The model under review builds one solid part; all positions refer to its coordinate system, in mm. A direction names the side the tool comes from. Round coordinates to 2 decimals unless told otherwise and drop trailing zeros. Order: outer loops, then holes, each group sorted by start corner. A loop starts at its lowest first (then second) coordinate and runs counter-clockwise, first axis right, second up. Notation, with made-up numbers: (85.25, 39.25) -> (106.25, 39.25) arc R12 cw to (106.25, 54.25) -> close; hole circle Ø6 at (10.5, 52). An arc over 180 degrees is marked (long way). Use a Markdown table: item, result. Add a question column.
Autodesk Inventor part; units mm, degrees
ref_plane "YZ Plane" through (0, 0, 0) normal (1, 0, 0) x (0, 1, 0)
ref_plane "XZ Plane" through (0, 0, 0) normal (0, 1, 0) x (-1, 0, 0)
ref_plane "XY Plane" through (0, 0, 0) normal (0, 0, 1) x (1, 0, 0)
sketch "Sketch1" plane through (0, 0, 0) normal (1, 0, 0) x (0, 1, 0)
  line L0 (0, 0) -> (100, 0)
  line L1 (100, 0) -> (100, -11)
  line L2 (100, -11) -> (0, -11)
  line L3 (0, -11) -> (0, 0)
  line L4 (60, -11) -> (40, -11)
  line L5 (40, -11) -> (40, -21)
  line L6 (40, -21) -> (60, -21)
  line L7 (60, -21) -> (60, -11)
  line L8 (0, -11) -> (100, -11)
  line L9 (100, -11) -> (100, -5)
  line L10 (100, -5) -> (0, -5)
  line L11 (0, -5) -> (0, -11)
  circle A0 centre (39, -12) radius 2.5
  line L12 (37.2322, -10.2322) -> (40.7678, -13.7678) construction
  circle A1 centre (61, -12) radius 2.5
  line L13 (62.7678, -10.2322) -> (59.2322, -13.7678) construction
  point P0 (0, -5)
  point P1 (60, -14.2913)
  point P2 (63.2913, -11)
  point P3 (36.7087, -11)
  point P4 (40, -14.2913)
  dimension "d1" = 11
  dimension "d2" = 100
  dimension "d3" = 10
  dimension "d4" = 20
  dimension "d5" = 40
  dimension "d7" = 6
  dimension "d31" = 5
  dimension "d32" = 45
  dimension "d33" = 1
  dimension "d34" = 1
  dimension "d35" = 5
  dimension "d36" = 45
  dimension "d37" = 1
  dimension "d38" = 1
revolve "Revolution1" add sketch "Sketch1" angle 360 about axis through (0, 0, 0) along (0, 1, 0) contours L10 L1 L2 A1 A0 L3 | L2 A1 L7 L6 L5 A0
sketch "Sketch2" plane through (0, 0, 0) normal (1, 0, 0) x (0, 1, 0)
  circle A0 centre (87, 0) radius 2
  line L0 (100, 11) -> (100, -11)
  point P0 (0, 0)
  dimension "d8" = 4
  dimension "d9" = 13
extrude "Extrusion1" cut sketch "Sketch2" along normal through all both and the other way through all
sketch "Sketch3" plane through (0, 0, 0) normal (0, 0, 1) x (1, 0, 0)
  circle A0 centre (0, 87) radius 2
  line L0 (-11, 100) -> (11, 100)
  point P0 (0, 0)
  dimension "d12" = 13
  dimension "d13" = 4
extrude "Extrusion2" cut sketch "Sketch3" against normal through all both and the other way through all
sketch "Sketch4" plane through (0, 0, 0) normal (0, -1, 0) x (1, 0, 0)
  circle A0 centre (0, 0) radius 9
  line L0 (-9, 0) -> (-11, 0)
  circle A1 centre (0, 0) radius 11
  line L1 (0, 9) -> (0, 11)
  line L2 (9, 0) -> (11, 0)
  line L3 (0, -9) -> (0, -11)
  line L4 (-4.5, -7.7942) -> (-5.5, -9.5263)
  line L5 (-7.7942, -4.5) -> (-9.5263, -5.5)
  line L6 (-7.7942, 4.5) -> (-9.5263, 5.5)
  line L7 (-4.5, 7.7942) -> (-5.5, 9.5263)
  line L8 (4.5, 7.7942) -> (5.5, 9.5263)
  line L9 (7.7942, 4.5) -> (9.5263, 5.5)
  line L10 (7.7942, -4.5) -> (9.5263, -5.5)
  line L11 (4.5, -7.7942) -> (5.5, -9.5263)
  dimension "d21" = 18
  dimension "d22" = 30
  dimension "d23" = 30
  dimension "d24" = 30
  dimension "d25" = 30
extrude "Extrusion3" cut sketch "Sketch4" against normal blind 30 contours A0 L9 A1 L2 | L10 A1 L11 A0 | A0 L1 A1 L8 | L3 A1 L4 A0 | A0 L6 A1 L7 | L5 A1 L0 A0
equation "\"d34\" = d33"
equation "\"d38\" = d37"
equation "\"d23\" = d22"
equation "\"d24\" = d22"
equation "\"d25\" = d22"
properties part number "shaft"
Q1. Mouldability with a two-part tool opening along X and no side actions: class faces 1 (the flat face through (14, 60, -4)), 2 (the cylindrical face through (0.923, 85.226, 7.836)), 3 (the cylindrical face through (-4.213, 81.389, -10.161)), 4 (the cylindrical face through (-6.34, 14.79, 6.39)) as pulls with the +X half, pulls with the -X half, needs draft (parallel to the pull), parting line crosses it, or undercut.
Q2. Add section C-C (y = 53). Write out the cut boundary in (x, z).
Q3. Add section B-B (y = 87). Write out the cut boundary in (x, z).
Q4. Add section A-A (y = 11.5). Write out the cut boundary in (x, z).
Q5. Wall thickness on line 1 (X direction, y = 36, z = 0); line 2 (Y direction, x = 6.75, z = 0); line 3 (Z direction, x = 19.5, y = 59): over which ranges is each line inside the solid? List them lowest first. Write a range as [from, to].
Q6. Machinability: for faces 5 (the cylindrical face through (-8.7, 14.8, -2.3)), 6 (the flat face through (0, 15, 10)), 7 (the flat face through (14, 40, -4)), 8 (the cylindrical face through (8.7, 14.8, 2.3)), which of the approach directions +Z, -Z, +X, -X, +Y, -Y give a long, thin tool a straight path to every point of the face, cutting with its end or side? Answer none if there is none.
Q7. Insertion check: pin 1 (3 mm diameter, centred on y = 87, z = 0, fed in from -X); pin 2 (1.6 mm diameter, centred on x = 9.5, y = 20.5, fed in from +Z); pin 3 (6 mm diameter, centred on x = -16, y = 43.5, fed in from +Z); pin 4 (0.6 mm diameter, centred on y = 12.5, z = -10, fed in from -X). Each pin has a flat end and moves straight along its axis. Give the tip position at first contact, or say it passes through.
Report:
| question | item | result |
|---|---|---|
| 1 | face 1 | needs draft |
| 1 | face 2 | undercut |
| 1 | face 3 | parting line crosses it |
| 1 | face 4 | undercut |
| 2 | outline | circle Ø42 at (0, 0); hole circle Ø10 at (0, 0) |
| 3 | outline | (-10.82, -2) arc R11 ccw to (-2, -10.82) -> (-2, -4.58) arc R5 cw to (-4.58, -2) -> close; (-10.82, 2) -> (-4.58, 2) arc R5 cw to (-2, 4.58) -> (-2, 10.82) arc R11 ccw to start; (2, -10.82) arc R11 ccw to (10.82, -2) -> (4.58, -2) arc R5 cw to (2, -4.58) -> close; (2, 4.58) arc R5 cw to (4.58, 2) -> (10.82, 2) arc R11 ccw to (2, 10.82) -> close |
| 4 | outline | (-11, 0) -> (-9, 0) arc R9 ccw to (-7.79, -4.5) -> (-9.53, -5.5) arc R11 ccw to (-5.5, -9.53) -> (-4.5, -7.79) arc R9 ccw to (0, -9) -> (0, -11) arc R11 ccw to (5.5, -9.53) -> (4.5, -7.79) arc R9 ccw to (7.79, -4.5) -> (9.53, -5.5) arc R11 ccw to (11, 0) -> (9, 0) arc R9 ccw to (7.79, 4.5) -> (9.53, 5.5) arc R11 ccw to (5.5, 9.53) -> (4.5, 7.79) arc R9 ccw to (0, 9) -> (0, 11) arc R11 ccw to (-5.5, 9.53) -> (-4.5, 7.79) arc R9 ccw to (-7.79, 4.5) -> (-9.53, 5.5) arc R11 ccw to start; hole circle Ø10 at (0, 0) |
| 5 | line 1 | x = [-11, -5], [5, 11] |
| 5 | line 2 | y = [0, 85], [89, 100] |
| 5 | line 3 | z = [-7.79, 7.79] |
| 6 | face 5 | -X, -Y |
| 6 | face 6 | +Z, -Y |
| 6 | face 7 | -Y |
| 6 | face 8 | +X, -Y |
| 7 | pin 1 | passes through |
| 7 | pin 2 | stops at z = 6.73 |
| 7 | pin 3 | stops at z = 16.49 |
| 7 | pin 4 | stops at x = 0 |
